Check sheet for the modelled part. Datum: model origin and axes. Units: mm. A direction names the side the tool comes from. Round coordinates to 2 decimals unless told otherwise and drop trailing zeros. Write each loop counter-clockwise with the first axis right and the second up, starting at its lowest first coordinate (ties: lowest second). Pieces come first, ordered by that corner, then holes.
Item 1: Cross-section at A-A on z = 1.25. Count the separate pieces of the cut face and the enclosed holes in it, plus the area to 3 significant figures.
Item 2: Material ranges on line 1 (Y direction, x = 33, z = 5); line 2 (Y direction, x = 57.15, z = 2); line 3 (X direction, y = 51, z = 6.25), recorded low to high.
Item 3: Tool access check on faces 5 (the flat face through (-16.13, -15.27, 3.13)), 6 (the cylindrical face through (-2.902, 47.662, 3.131)), 7 (the cylindrical face through (19.858, 18.275, 3.131)), 8 (the flat face through (7, 110, 0)), 9 (the cylindrical face through (-4.14, 201.63, 3.13)). Record the directions out of +Z, -Z, +X, -X, +Y, -Y that give a thin tool (end or side, any length) a straight path to the whole face; none if there is none.
Item 4: Cross-section at B-B on y = 177. Enter the section's corners in (x, z), plus the area to 3 significant figures.
Item 5: Cross-section at C-C on y = 46. Enter the section's corners in (x, z).
Item 6: Go/stop test with flat-tipped pins: pin 1 Ø3 at (x, z) = (36, 2.5) entering from -Y; pin 2 Ø1.5 at (x, z) = (-12, 2) entering from -Y; pin 3 Ø1.9 at (y, z) = (-3, 3.5) entering from +X. Record where each tip stops, or that it passes through.
Item 7: Release check for a two-part mould opening along X. For faces 1 (the cylindrical face through (7.77, 11.134, 3.131)), 2 (the flat face through (42, 190.5, 3)), 3 (the cylindrical face through (-1.36, 188.31, 3.13)), 4 (the cylindrical face through (26.6, 11.3, 3.1)) record: +X half, -X half, draft (parallel to the pull), parting line (faces both ways), or undercut.
from build123d import *

# Parameters (mm, degrees)
SKETCH1_R           = 2.38125
BOSS_EXTRUDE1_DEPTH = 6.35


with BuildPart() as part:
    # Sketch1 → Boss-Extrude1 (new body)
    with BuildSketch(Plane.XY):
        with BuildLine():
            Line((0, 80.374326863), (0, 184.169856168))
            ThreePointArc((0, 184.169856168), (-1.399519198, 188.364212997), (-5.037259615, 190.877801635))
            ThreePointArc((-5.037259615, 190.877801635), (-11.811326602, 201.366372539), (-2.38125, 209.55))
            Line((-2.38125, 209.55), (57.15, 209.55))
            ThreePointArc((57.15, 209.55), (66.675, 200.025), (57.15, 190.5))
            Line((57.15, 190.5), (26.035, 190.5))
            ThreePointArc((26.035, 190.5), (21.095859133, 188.454140867), (19.05, 183.515))
            Line((19.05, 183.515), (19.05, 21.407957037))
            ThreePointArc((19.05, 21.407957037), (19.880728328, 18.234450269), (22.159817881, 15.875))
            ThreePointArc((22.159817881, 15.875), (26.628620925, 11.248626923), (28.2575, 5.026064633))
            Line((28.2575, 5.026064633), (28.2575, -23.8125))
            ThreePointArc((28.2575, -23.8125), (25.87625, -26.19375), (23.495, -23.8125))
            Line((23.495, -23.8125), (23.495, -6.477))
            ThreePointArc((23.495, -6.477), (21.597930622, -1.897069378), (17.018, 0))
            Line((17.018, 0), (-2.638551939, 0))
            ThreePointArc((-2.638551939, 0), (-9.136828191, -2.048898632), (-13.284704491, -7.45451627))
            Line((-13.284704491, -7.45451627), (-19.055961271, -23.310913955))
            ThreePointArc((-19.055961271, -23.310913955), (-23.125399297, -25.208524071), (-25.023009413, -21.139086045))
            Line((-25.023009413, -21.139086045), (-11.205694737, 16.823674026))
            ThreePointArc((-11.205694737, 16.823674026), (-2.822866527, 48.108814817), (0, 80.374326863))
        make_face()
        with Locations((9.525, 9.525)):
            Circle(SKETCH1_R, mode=Mode.SUBTRACT)
        with Locations((9.525, 200.025)):
            Circle(SKETCH1_R, mode=Mode.SUBTRACT)
        with Locations((21.43125, 200.025)):
            Circle(SKETCH1_R, mode=Mode.SUBTRACT)
        with Locations((-2.38125, 200.025)):
            Circle(SKETCH1_R, mode=Mode.SUBTRACT)
        with Locations((33.3375, 200.025)):
            Circle(SKETCH1_R, mode=Mode.SUBTRACT)
        with Locations((57.15, 200.025)):
            Circle(SKETCH1_R, mode=Mode.SUBTRACT)
        with Locations((45.24375, 200.025)):
            Circle(SKETCH1_R, mode=Mode.SUBTRACT)
    extrude(amount=BOSS_EXTRUDE1_DEPTH)


solid = part.part
Response values:
1. separate pieces: 1
1. enclosed holes: 7
1. area: 5,860 mm2
2. line 1: y = 190.5 to 197.67, 202.38 to 209.55
2. line 2: y = 190.5 to 197.64, 202.41 to 209.55
2. line 3: x = -2.34 to 19.05
3. face 5: +Z, -Z, -Y
3. face 6: +Z, -Z, -X
3. face 7: +Z, -Z, +X
3. face 8: -Z, +X, -X, +Y, -Y
3. face 9: +Z, -Z
4. outline: (0, 0) - (19.05, 0) - (19.05, 6.35) - (0, 6.35) - close
4. area: 121 mm2
5. outline: (-3.21, 0) - (19.05, 0) - (19.05, 6.35) - (-3.21, 6.35) - close
6. pin 1: stops at y = 190.5
6. pin 2: stops at y = -6.22
6. pin 3: stops at x = 28.26
7. face 1: undercut
7. face 2: draft
7. face 3: -X half
7. face 4: +X half
